The listing builds one solid part. Answer for the finished solid, in the listing's coordinates (mm). A direction names the side the tool comes from. Coordinates: 2 decimals unless noted, no trailing zeros. Order: outer loops, then holes, each group sorted by start corner. A loop starts at its lowest first (then second) coordinate and runs counter-clockwise, first axis right, second up. Notation, with made-up numbers: (-17, 88.25) -> (5, 88.25) arc R18 cw to (5, 98.25) -> close; hole circle Ø10 at (78, -13). An arc over 180 degrees is marked (long way). One line per question, with ' | ' between items.
from build123d import *

# Parameters (mm, degrees)
BOSS_EXTRUDE1_DEPTH = 6.35
FILLET1_R           = 5
FILLET2_R           = 15
SKETCH4_R           = 2.75
CUT_EXTRUDE2_DEPTH  = 10
CUT_EXTRUDE3_REACH  = 48.24
SKETCH3_R           = 2.75


with BuildPart() as part:
    # Sketch1 → Boss-Extrude1 (new body)
    with BuildSketch(Plane.XY):
        with BuildLine():
            Line((0, 0), (-64, 0))
            Line((-64, 0), (-64, -12.552169744))
            ThreePointArc((-64, -12.552169744), (-70.352218413, -27.887781587), (-85.687830256, -34.24))
            Line((-85.687830256, -34.24), (-194.687830256, -34.24))
            Line((-194.687830256, -34.24), (-194.687830256, -46.24))
            Line((-194.687830256, -46.24), (-85.687830256, -46.24))
            ThreePointArc((-85.687830256, -46.24), (-61.866937038, -36.373062962), (-52, -12.552169744))
            Line((-52, -12.552169744), (-52, -8))
            Line((-52, -8), (0, -8))
            Line((0, -8), (0, 0))
        make_face()
    extrude(amount=BOSS_EXTRUDE1_DEPTH)

    # Fillet1
    fillet1_edges = [part.edges().sort_by_distance(p)[0] for p in [
        (-194.687830256, -46.24, 3.175),
        (-194.687830256, -34.24, 3.175),
        (-64, 0, 3.175),
    ]]
    fillet(fillet1_edges, radius=FILLET1_R)

    # Fillet2
    fillet2_edges = [part.edges().sort_by_distance(p)[0] for p in [
        (-52, -8, 3.175),
    ]]
    fillet(fillet2_edges, radius=FILLET2_R)

    # Sketch4 → Cut-Extrude2 (cut)
    with BuildSketch(Plane.XY.offset(6.35)):
        with Locations((-164.687830256, -40.24)):
            Circle(SKETCH4_R)
        with Locations((-114.687830256, -40.24)):
            Circle(SKETCH4_R)
        with Locations((-6.452530622, -4)):
            Circle(SKETCH4_R)
        with Locations((-28.952530622, -4)):
            Circle(SKETCH4_R)
        with Locations((-51.452530622, -4)):
            Circle(SKETCH4_R)
    extrude(amount=-CUT_EXTRUDE2_DEPTH, mode=Mode.SUBTRACT)

    # Sketch3 → Cut-Extrude3 (cut, up to next)
    with BuildSketch(Plane(origin=(0, 0, 0), x_dir=(1, 0, 0), z_dir=(0, 1, 0)), mode=Mode.PRIVATE) as cut_extrude3_sk1:
        with Locations((-13, 0)):
            Circle(SKETCH3_R)
    cut_extrude3_tool1 = extrude(cut_extrude3_sk1.sketch, amount=-CUT_EXTRUDE3_REACH, mode=Mode.PRIVATE) & part.part
    add(cut_extrude3_tool1.solids().sort_by_distance((-13, 0, 0))[0], mode=Mode.SUBTRACT)
    # Sketch3 → Cut-Extrude3 (cut, up to next)
    with BuildSketch(Plane(origin=(0, 0, 0), x_dir=(1, 0, 0), z_dir=(0, 1, 0)), mode=Mode.PRIVATE) as cut_extrude3_sk2:
        with Locations((-38, 0)):
            Circle(SKETCH3_R)
    cut_extrude3_tool2 = extrude(cut_extrude3_sk2.sketch, amount=-CUT_EXTRUDE3_REACH, mode=Mode.PRIVATE) & part.part
    add(cut_extrude3_tool2.solids().sort_by_distance((-38, 0, 0))[0], mode=Mode.SUBTRACT)


solid = part.part
Item 1: Each of these flat-tipped pins is pushed along its axis until it touches: pin 1 Ø2 at (y, z) = (-18, 1) entering from +X; pin 2 Ø3 at (x, z) = (-143.5, 3) entering from +Y; pin 3 Ø3 at (x, z) = (-24.5, 4) entering from -Y. Where does it stop, or does it pass through?
Computed values:
pin 1: stops at x = -51.88 | pin 2: stops at y = -34.24 | pin 3: stops at y = -8
Item 2: Section C-C, the plane x = -99 is taken. Give the vertices of the cut face in (y, z).
Computed values:
outline: (-46.24, 0) -> (-34.24, 0) -> (-34.24, 6.35) -> (-46.24, 6.35) -> close
Item 3: Find the intervals of material crossed by L1, parallel to X at y = -38, z = 3; L2, parallel to X at y = -41, z = 1; L3, parallel to X at y = -3, z = 0.5, in increasing order.
Computed values:
L1: x = -194.53 to -166.28, -163.09 to -116.28, -113.09 to -63.61 | L2: x = -194.69 to -167.33, -162.04 to -117.33, -112.04 to -67.64 | L3: x = -63.58 to -54.01, -48.89 to -40.7, -35.3 to -31.51, -26.39 to -15.7, -10.3 to -9.01, -3.89 to 0
Item 4: Section B-B, the plane z = 1 is taken. Count the separate pieces of the cut face and the enclosed holes in it, plus the area to 3 significant figures.
Computed values:
separate pieces: 3 | enclosed holes: 5 | area: 2,220 mm^2
Item 5: Section A-A, the plane x = -13 is taken. Give the vertices of the cut face in (y, z), plus the area to 3 significant figures.
Computed values:
outline: (-8, 2.75) -> (0, 2.75) -> (0, 6.35) -> (-8, 6.35) -> close | area: 28.8 mm^2
Item 6: For faces 1 (the face through (-7.049, -6.685, 3.219)), 2 (the face through (-137, -34.24, 3)), determine the directions among +Z, -Z, +X, -X, +Y, -Y from which every point of the face is accessible in a straight line to the end or side of a thin tool.
Computed values:
face 1: +Z, -Z | face 2: +Z, -Z, -X, +Y
Item 7: Determine the mould class of faces 3 (the face through (-112, -35, 0)), 4 (the face through (-138, -46.24, 3)), 5 (the face through (-26.41, -5.05, 3.22)) for opening direction Y: pulls with the +Y half, pulls with the -Y half, needs draft (parallel to the pull), parting line crosses it, or undercut.
Computed values:
face 3: needs draft | face 4: pulls with the -Y half | face 5: undercut
